Autodesk Inventor part; units mm, degrees
ref_plane "YZ Plane" through (0, 0, 0) normal (1, 0, 0) x (0, 1, 0)
ref_plane "XZ Plane" through (0, 0, 0) normal (0, 1, 0) x (-1, 0, 0)
ref_plane "XY Plane" through (0, 0, 0) normal (0, 0, 1) x (1, 0, 0)
sketch "Эскиз1" plane through (0, 0, 0) normal (0, 0, 1) x (1, 0, 0)
  arc A0 (-38.2043, 10.8524) -> (-38.2043, -10.8524) centre (-40, 0) ccw
  arc A1 (-10.8524, -38.2043) -> (10.8524, -38.2043) centre (0, -40) ccw
  arc A2 (10.8524, 38.2043) -> (-10.8524, 38.2043) centre (0, 40) ccw
  arc A3 (38.2043, -10.8524) -> (38.2043, 10.8524) centre (40, 0) ccw
  arc A4 (-38.2043, 10.8524) -> (-36.0537, 12.0056) centre (-37.8778, 12.8256) ccw
  arc A5 (-36.0537, -12.0056) -> (-38.2043, -10.8524) centre (-37.8778, -12.8256) ccw
  arc A6 (-10.8524, -38.2043) -> (-12.0056, -36.0537) centre (-12.8256, -37.8778) ccw
  arc A7 (12.0056, -36.0537) -> (10.8524, -38.2043) centre (12.8256, -37.8778) ccw
  arc A8 (38.2043, -10.8524) -> (36.0537, -12.0056) centre (37.8778, -12.8256) ccw
  arc A9 (36.0537, 12.0056) -> (38.2043, 10.8524) centre (37.8778, 12.8256) ccw
  arc A10 (10.8524, 38.2043) -> (12.0056, 36.0537) centre (12.8256, 37.8778) ccw
  arc A11 (-12.0056, 36.0537) -> (-10.8524, 38.2043) centre (-12.8256, 37.8778) ccw
  arc A12 (-12.0056, 36.0537) -> (-36.0537, 12.0056) centre (0, 0) ccw
  arc A13 (36.0537, 12.0056) -> (12.0056, 36.0537) centre (0, 0) ccw
  arc A14 (-36.0537, -12.0056) -> (-12.0056, -36.0537) centre (0, 0) ccw
  arc A15 (12.0056, -36.0537) -> (36.0537, -12.0056) centre (0, 0) ccw
  dimension "d87" = 22
  dimension "d88" = 22
  dimension "d89" = 22
  dimension "d90" = 22
  dimension "d91" = 40
  dimension "d92" = 40
  dimension "d93" = 40
  dimension "d94" = 40
  dimension "d95" = 4
  dimension "d96" = 4
  dimension "d97" = 4
  dimension "d98" = 4
  dimension "d99" = 4
  dimension "d100" = 4
  dimension "d101" = 4
  dimension "d102" = 4
  dimension "d103" = 38
  dimension "d104" = 38
  dimension "d105" = 38
  dimension "d106" = 38
  dimension "d107" = 37.8778
  dimension "d108" = 37.8778
  dimension "d109" = 37.8778
  dimension "d110" = 37.8778
  dimension "d111" = 37.8778
  dimension "d112" = 37.8778
  dimension "d113" = 37.8778
  dimension "d114" = 37.8778
extrude "Выдавливание1" add sketch "Эскиз1" along normal blind 20
sketch "Эскиз4" plane through (0, 0, 0) normal (0, 1, 0) x (-1, 0, 0)
  line L0 (0, 0) -> (29, 0)
  line L1 (0, 10) -> (15, 10)
  line L2 (15, 10) -> (29, 0)
  line L3 (0, 10) -> (0, 0)
  line L4 (11, 0) -> (-11, 0)
  line L5 (0, -4) -> (0, 24)
  point P0 (10.8524, 0)
  point P1 (-10.8524, 0)
  dimension "d115" = 29
  dimension "d116" = 15
  dimension "d117" = 10
revolve "Вращение4" cut sketch "Эскиз4" angle 360 about axis through (0, 0, -10) along (0, 0, 1)
sketch "Эскиз5" plane through (0, 0, 0) normal (0, 1, 0) x (-1, 0, 0)
  line L0 (-51, 0) -> (-51, 20)
  line L1 (-51, 10) -> (-29, 10)
  line L2 (-29, 10) -> (-15, 20)
  line L3 (-15, 20) -> (-51, 20)
  line L4 (-12.0056, 20) -> (-36.0537, 20)
  line L5 (-15, 10) -> (-29, 0)
  line L6 (-38.2043, 0) -> (-51, 0)
  line L7 (0, -4) -> (0, 24)
  point P0 (0, 0)
  dimension "d120" = 10
  dimension "d122" = 29
revolve "Вращение5" cut sketch "Эскиз5" angle 360 about axis through (0, 0, -10) along (0, 0, 1)
sketch "Эскиз6" plane through (0, -40, 10) normal (0, 0, 1) x (1, 0, 0)
  circle A0 centre (0, 0) radius 7
  circle A1 centre (-40, 40) radius 7
  circle A2 centre (0, 80) radius 7
  circle A3 centre (40, 40) radius 7
  point P0 (0, 40)
  dimension "d125" = 40
  dimension "d126" = 40
  dimension "d127" = 40
  dimension "d128" = 40
  dimension "d129" = 14
  dimension "d130" = 14
  dimension "d131" = 14
  dimension "d132" = 14
hole "Отверстие1" at (0, -40, 10) at (-40, 0, 10) at (40, 0, 10) at (0, 40, 10) direction (0, 0, -1) diameter 14 depth 10
Can you work these out from the model? Positions are in its coordinate system, mm. A direction names the side the tool comes from. Coordinates: 2 decimals unless noted, no trailing zeros. Order: outer loops, then holes, each group sorted by start corner. A loop starts at its lowest first (then second) coordinate and runs counter-clockwise, first axis right, second up. Notation, with made-up numbers: (65.25, 68.25) - (71.25, 68.25) arc R12 ccw to (71.25, 91.25) - close; hole circle Ø1 at (-40, 64). An arc over 180 degrees is marked (long way). Answer as a JSON object with one key per item and string values. Group by question number.
Q1. We'd pull the mould along X, two halves only. Please class faces 4 (the face through (11.701, 10.73, 9.374)), 5 (the face through (-3.442, 15.498, 19.374)), 6 (the face through (26.695, 27.044, 4.93)): +X half, -X half, draft (parallel to the pull), parting line (faces both ways), or undercut.
Q2. Imagine slicing it at B-B (y = 0). Please give me the cut outline in (x, z), and give its area (3 significant figures).
Q3. I need wall thicknesses on line 1 (X direction, y = 40, z = 8.25); line 2 (Z direction, x = 34, y = -7.5). Which ranges of each line are inside material? Lowest first, please. Write a range as from..to.
Q4. Will these pins go through, and if not, where does the flat tip stop? P1, Ø15, axis at x = -6.5, y = -5, coming from the -Z side; P2, Ø3, axis at x = -4.5, y = -8, coming from the -Z side; P3, Ø22.5, axis at x = 0, y = -40, coming from the +Z side; P4, Ø16, axis at x = 0, y = 40, coming from the -Z side.
Q5. Imagine slicing it at A-A (x = 40). Please give me the cut outline in (y, z), and give its area (3 significant figures).
Q6. On a 3-axis mill with a long thin cutter (end or side, diameter ignored), from which of +Z, -Z, +X, -X, +Y, -Y can I reach the whole of each face in a straight line? I mean faces 1 (the face through (-26.695, -27.044, 4.93)), 2 (the face through (0, 0, 10)), 3 (the face through (-23, -19, 10)). Say none if no direction works.
Determined:
{
 "1": {"face 4": "undercut", "face 5": "parting line", "face 6": "+X half"},
 "2": {"outline": "(-51, 0) - (-47, 0) - (-47, 10) - (-51, 10) - close; (-33, 0) - (-29, 0) - (-15, 10) - (15, 10) - (29, 0) - (33, 0) - (33, 10) - (29, 10) - (15, 20) - (-15, 20) - (-29, 10) - (-33, 10) - close; (47, 0) - (51, 0) - (51, 10) - (47, 10) - close", "area": "740 mm2"},
 "3": {"line 1": "x = -11..-7, 7..11", "line 2": "z = 0..10"},
 "4": {"P1": "stops at z = 9.5", "P2": "stops at z = 10", "P3": "stops at z = 10.18", "P4": "stops at z = 0"},
 "5": {"outline": "(-11, 0) - (-7, 0) - (-7, 10) - (-11, 10) - close; (7, 0) - (11, 0) - (11, 10) - (7, 10) - close", "area": "80.0 mm2"},
 "6": {"face 1": "+Z, -Z, -X, -Y", "face 2": "-Z", "face 3": "+Z"}
}
